Geometry check sheet. Reference: drawing and pictorial views, mm from the part's lowest x, y, z. A direction names the side the tool comes from. Give positions to 0.01 mm unless a question says otherwise; leave off trailing zeros. Order: outer loops, then holes, each group sorted by start corner. A loop starts at its lowest first (then second) coordinate and runs counter-clockwise, first axis right, second up. Notation, with made-up numbers: (66, 8.25) - (111, 8.25) arc R14 cw to (111, 31.25) - close; hole circle Ø6 at (-11, 43.5). An arc over 180 degrees is marked (long way). Answer in a Markdown table with one row per item.
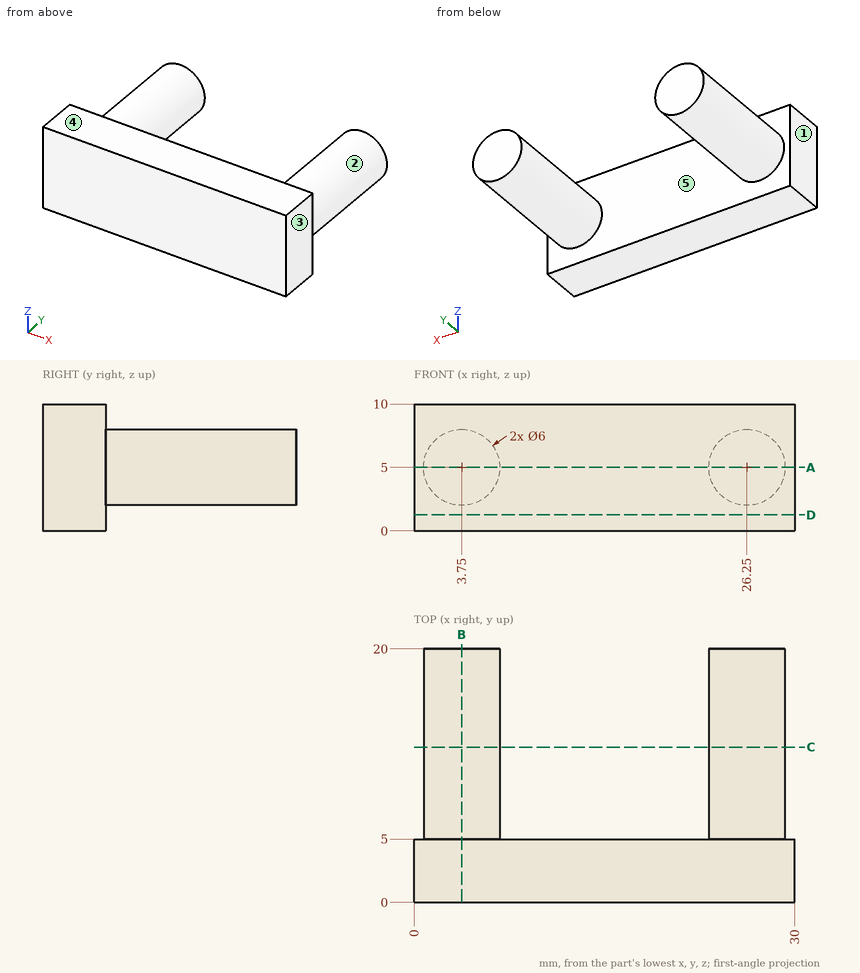
(1) Cross-section at C-C, the plane y = 12.25. Record the cut outline in (x, z).
Geometry says:
| item | result |
|---|---|
| outline | circle Ø6 at (3.75, 5); circle Ø6 at (26.25, 5) |
(2) Mould release check, pull along X, two halves, no side actions. Record for the marked faces 1, 2 and 3: pulls with the +X half, pulls with the -X half, needs draft (parallel to the pull), parting line crosses it, or undercut.
Geometry says:
| item | result |
|---|---|
| face 1 | pulls with the -X half |
| face 2 | undercut |
| face 3 | pulls with the +X half |
(3) Cross-section at D-D, the plane z = 1.25. Record the cut outline in (x, y), then the cut area to 3 significant figures.
Geometry says:
| item | result |
|---|---|
| outline | (0, 0) - (30, 0) - (30, 5) - (0, 5) - close |
| area | 150 mm² |
(4) Access from +Z, -Z, +X, -X, +Y, -Y to the whole of each face (thin tool, end or side, straight path). Record for the marked faces 4 and 5.
Geometry says:
| item | result |
|---|---|
| face 4 | +Z, +X, -X, +Y, -Y |
| face 5 | +Y |
(5) Cross-section at B-B, the plane x = 3.75. Record the cut outline in (y, z).
Geometry says:
| item | result |
|---|---|
| outline | (0, 0) - (5, 0) - (5, 2) - (20, 2) - (20, 8) - (5, 8) - (5, 10) - (0, 10) - close |
(6) Gauge pin test, flat ends, axial feed: P1, Ø1, axis at y = 13.5, z = 7.5, coming from the -X side; P2, Ø1.5, axis at y = 11.5, z = 3.5, coming from the +X side; P3, Ø5, axis at x = 16.5, z = 5, coming from the +Y side; P4, Ø2, axis at y = 3, z = 6, coming from the -X side. Record the tip position at first contact, or that the pin passes through.
Geometry says:
| item | result |
|---|---|
| P1 | x = 1.51 |
| P2 | x = 29.15 |
| P3 | y = 5 |
| P4 | x = 0 |
(7) Thickness scan on L1, parallel to Y at x = 12, z = 5.5; L2, parallel to X at y = 9, z = 3; L3, parallel to X at y = 15.25, z = 3.5. Record the ranges inside material, lowest first.
Geometry says:
| item | result |
|---|---|
| L1 | 0 to 5 |
| L2 | 1.51 to 5.99, 24.01 to 28.49 |
| L3 | 1.15 to 6.35, 23.65 to 28.85 |
(8) Cross-section at A-A, the plane z = 5. Record the cut outline in (x, y).
Geometry says:
| item | result |
|---|---|
| outline | (0, 0) - (30, 0) - (30, 5) - (29.25, 5) - (29.25, 20) - (23.25, 20) - (23.25, 5) - (6.75, 5) - (6.75, 20) - (0.75, 20) - (0.75, 5) - (0, 5) - close |
